CAD build for the part. Positions are in the model's coordinates, mm. A direction names the side the tool comes from. Give positions to 0.01 mm unless a question says otherwise; leave off trailing zeros. Write each loop counter-clockwise with the first axis right and the second up, starting at its lowest first coordinate (ties: lowest second). Pieces come first, ordered by that corner, then holes. Notation, with made-up numbers: (-39.75, 26.25) - (0.25, 26.25) arc R16 ccw to (0.25, 31.25) - close; hole circle Ø6 at (-30.5, -15.75). An arc over 180 degrees is marked (long way). Answer as a JSON object with one key per item and string values.
from build123d import *

# Parameters (mm, degrees)
SKETCH_1_W           = 20
SKETCH_1_H           = 60
EXTRUDE_1_DEPTH      = 20
FILLET_1_R           = 2
SKETCH_2_W           = 16
SKETCH_2_H           = 1.155895232
EXTRUDE_2_DEPTH      = 0.5
EXTRUDE_3_DEPTH      = 2.1
EXTRUDE_3_DEPTH_BACK = 18.2
SKETCH_4_W           = 0.476897723
SKETCH_4_H           = 2.004187554
SKETCH_4_W_2         = 0.424555406
EXTRUDE_4_DEPTH      = 0.1
EXTRUDE_5_DEPTH      = 6.83
CUT_EXTRUDE_1_DEPTH  = 6.83
SKETCH_7_W           = 11.171140339
SKETCH_7_H           = 6.83
EXTRUDE_6_DEPTH      = 0.1
FILLET_5_R           = 0.5


with BuildPart() as part:
    # 草图1 → 凸台-拉伸1 (new body)
    with BuildSketch(Plane(origin=(0, 0, 0), x_dir=(0, 0, -1), z_dir=(1, 0, 0))):
        Rectangle(SKETCH_1_W, SKETCH_1_H)
    extrude(amount=EXTRUDE_1_DEPTH)

    # 圆角1
    fillet_1_edges = [part.edges().sort_by_distance(p)[0] for p in [
        (20, 0, 10),
        (20, -30, 0),
        (20, 0, -10),
        (0, -30, 0),
        (0, 0, 10),
        (0, 30, 0),
        (0, 0, -10),
        (10, -30, -10),
        (10, -30, 10),
        (10, 30, 10),
        (10, 30, -10),
        (20, 30, 0),
    ]]
    fillet(fillet_1_edges, radius=FILLET_1_R)

    # 草图2 → 凸台-拉伸2 (add)
    with BuildSketch(Plane.XY.offset(10)):
        with Locations((10, 0.577947616)):
            Rectangle(SKETCH_2_W, SKETCH_2_H)
    extrude(amount=EXTRUDE_2_DEPTH)

    # 草图3 → 凸台-拉伸3 (add, two sides: drawn at the far end of the back side and taken through both)
    with BuildSketch(Plane(origin=(18, 0, 0), x_dir=(0, 0, -1), z_dir=(1, 0, 0)).offset(-EXTRUDE_3_DEPTH_BACK)):
        Polygon((-10.5, 1.155895232), (-10.5, 4.667192464), (10.350971517, 4.667192464), (10.350971517, -2.166522321), (-10.5, -2.166522321), align=None)
    extrude(amount=EXTRUDE_3_DEPTH + EXTRUDE_3_DEPTH_BACK)

    # 草图4 → 凸台-拉伸4 (add)
    with BuildSketch(Plane.ZY):
        with Locations((-5.238448862, 5.669286241)):
            Rectangle(SKETCH_4_W, SKETCH_4_H)
        with Locations((5.212277703, 5.669286241)):
            Rectangle(SKETCH_4_W_2, SKETCH_4_H)
    extrude(amount=EXTRUDE_4_DEPTH)

    # 草图5 → 凸台-拉伸5 (add)
    with BuildSketch(Plane.XZ.offset(2.166522321)):
        Polygon((-0.2, -10.350971517), (-0.2, 8), (-4.654545455, 8), (-10, 5), (-10, 0), (-10, -6.171140339), align=None)
        Polygon((-4.654545455, 8), (-0.2, 8), (-0.2, 10.5), align=None)
    extrude(amount=-EXTRUDE_5_DEPTH)

    # 草图6 → 切除-拉伸1 (cut)
    with BuildSketch(Plane.XZ.offset(2.166522321)):
        Polygon((-9.707704369, -5.877282194), (-0.2, -10.073184662), (-0.2, 10.062586421), (-9.707704369, 4.749296883), align=None)
    extrude(amount=-CUT_EXTRUDE_1_DEPTH, mode=Mode.SUBTRACT)

    # 草图7 → 凸台-拉伸6 (add)
    with BuildSketch(Plane.ZY.offset(10)):
        with Locations((-0.58557017, 1.248477679)):
            Rectangle(SKETCH_7_W, SKETCH_7_H)
    extrude(amount=EXTRUDE_6_DEPTH)

    # 圆角5
    fillet_5_edges = [part.edges().sort_by_distance(p)[0] for p in [
        (20.1, 1.250335071, 10.5),
        (20.1, 1.250335071, -10.350971517),
    ]]
    fillet(fillet_5_edges, radius=FILLET_5_R)


solid = part.part
Item 1: Mould opens along X. For faces 5 (the cylindrical face through (10.11, 29.4, -9.43)), 6 (the flat face through (-9.708, 1, 0)), 7 (the cylindrical face through (0.6, 16.5, 9.43)) say: +X half, -X half, draft (parallel to the pull), parting line (faces both ways), or undercut.
Entries:
{"face 5": "draft", "face 6": "undercut", "face 7": "-X half"}
Item 2: Cut at C-C (x = 11.5). Give the cut face in (y, z).
Entries:
{"outline": "(-30, -8) arc R2 ccw to (-28, -10) - (-2.17, -10) - (-2.17, -10.35) - (4.67, -10.35) - (4.67, -10) - (28, -10) arc R2 ccw to (30, -8) - (30, 8) arc R2 ccw to (28, 10) - (4.67, 10) - (4.67, 10.5) - (-2.17, 10.5) - (-2.17, 10) - (-28, 10) arc R2 ccw to (-30, 8) - close"}
Item 3: Flat gauge pins, fed straight in: P1, Ø1.5, axis at x = -2, z = -6, coming from the -Y side; P2, Ø5, axis at y = -18, z = 3, coming from the +X side; P3, Ø17.5, axis at x = 10.5, y = 13.5, coming from the +Z side; P4, Ø5, axis at y = -16.5, z = -2, coming from the -X side. Where does each tip first touch, or does it go through?
Entries:
{"P1": "through", "P2": "x = 20", "P3": "z = 10", "P4": "x = 0"}
Item 4: Probe line 1 (X direction, y = 17.5, z = -7.5); line 2 (Z direction, x = 15.5, y = 18); line 3 (Z direction, x = 1, y = -24). List the from-to ranges inside material, lowest first. Write a range as from..to.
Entries:
{"line 1": "0..20", "line 2": "-10..10", "line 3": "-9.73..9.73"}
Item 5: Cut at D-D (z = -6.75). Give the cut face in (x, y), and give its area (3 significant figures).
Entries:
{"outline": "(-8.64, -2.17) - (-7.73, -2.17) - (-7.73, 4.66) - (-8.64, 4.66) - close; (-0.2, -2.17) - (0, -2.17) - (0, -28) arc R2 ccw to (2, -30) - (18, -30) arc R2 ccw to (20, -28) - (20, -2.17) - (20.1, -2.17) - (20.1, 4.67) - (20, 4.67) - (20, 28) arc R2 ccw to (18, 30) - (2, 30) arc R2 ccw to (0, 28) - (0, 4.67) - (-0.2, 4.67) - close", "area": "1,200 mm2"}
Item 6: Cut at B-B (y = 10). Give the cut face in (x, z).
Entries:
{"outline": "(0, -8) arc R2 ccw to (2, -10) - (18, -10) arc R2 ccw to (20, -8) - (20, 8) arc R2 ccw to (18, 10) - (2, 10) arc R2 ccw to (0, 8) - close"}
Item 7: Which spindle directions (+Z, -Z, +X, -X, +Y, -Y) get a long thin tool onto all of the face, cutting with end or side? Do faces 1 (the cylindrical face through (19.4, 16.5, 9.43)), 2 (the flat face through (20, -15, 0)), 3 (the flat face through (0, -15, 0)), 4 (the cylindrical face through (0.6, -14.9, -9.43)). Say none if no direction does.
Entries:
{"face 1": "+Z, +X, +Y", "face 2": "+Z, -Z, +X, -Y", "face 3": "+Z, -Z, -X, -Y", "face 4": "-Z, -X, -Y"}
Item 8: Cut at A-A (z = -1.5). Give the cut face in (x, y), and give its area (3 significant figures).
Entries:
{"outline": "(-10.1, -2.17) - (-9.71, -2.17) - (-9.71, 4.66) - (-10.1, 4.66) - close; (-0.2, -2.17) - (0, -2.17) - (0, -28) arc R2 ccw to (2, -30) - (18, -30) arc R2 ccw to (20, -28) - (20, -2.17) - (20.1, -2.17) - (20.1, 4.67) - (20, 4.67) - (20, 28) arc R2 ccw to (18, 30) - (2, 30) arc R2 ccw to (0, 28) - (0, 4.67) - (-0.2, 4.67) - close", "area": "1,200 mm2"}
